```python
from build123d import *

# Parameters (mm, degrees)
SKETCH2_W             = 120
SKETCH2_H             = 160
SKETCH2_R             = 14.002160315
SKETCH2_R_2           = 1.35
BOSS_EXTRUDE1_DEPTH   = 4
SKETCH4_R             = 1.75
CUT_EXTRUDE1_DEPTH    = 4
SKETCH6_R             = 2.075123243
SKETCH6_R_2           = 1.889494125
BOSS_EXTRUDE2_DEPTH   = 4
BOSS_EXTRUDE2_2_DEPTH = 4
BOSS_EXTRUDE2_3_DEPTH = 4
BOSS_EXTRUDE2_4_DEPTH = 4


with BuildPart() as part:
    # Sketch2 → Boss-Extrude1 (new body)
    with BuildSketch(Plane(origin=(0, 0, 0), x_dir=(1, 0, 0), z_dir=(0, 1, 0))):
        Rectangle(SKETCH2_W, SKETCH2_H)
        Circle(SKETCH2_R, mode=Mode.SUBTRACT)
        with Locations((-28.228110793, -22.694220691)):
            Circle(SKETCH2_R_2, mode=Mode.SUBTRACT)
        with Locations((-24.5, -29)):
            Circle(SKETCH2_R_2, mode=Mode.SUBTRACT)
        with Locations((24.5, -29)):
            Circle(SKETCH2_R_2, mode=Mode.SUBTRACT)
        with Locations((29.771889207, -22.694220691)):
            Circle(SKETCH2_R_2, mode=Mode.SUBTRACT)
        with Locations((29.771889207, 26.305779309)):
            Circle(SKETCH2_R_2, mode=Mode.SUBTRACT)
        with Locations((24.5, 29)):
            Circle(SKETCH2_R_2, mode=Mode.SUBTRACT)
        with Locations((-28.228110793, 26.305779309)):
            Circle(SKETCH2_R_2, mode=Mode.SUBTRACT)
        with Locations((-24.5, 29)):
            Circle(SKETCH2_R_2, mode=Mode.SUBTRACT)
    extrude(amount=BOSS_EXTRUDE1_DEPTH)

    # Sketch4 → Cut-Extrude1 (cut)
    with BuildSketch(Plane(origin=(0, 4, 0), x_dir=(1, 0, 0), z_dir=(0, 1, 0))):
        with Locations((-6, 74.910885073)):
            Circle(SKETCH4_R)
        with Locations((-6, 69.410885073)):
            Circle(SKETCH4_R)
        with Locations((-55.5, 69.410885073)):
            Circle(SKETCH4_R)
        with Locations((-55.5, 74.910885073)):
            Circle(SKETCH4_R)
        with Locations((55.5, 74.910885073)):
            Circle(SKETCH4_R)
        with Locations((55.5, 69.410885073)):
            Circle(SKETCH4_R)
        with Locations((6, 69.410885073)):
            Circle(SKETCH4_R)
        with Locations((6, 74.910885073)):
            Circle(SKETCH4_R)
        with Locations((-6, -69)):
            Circle(SKETCH4_R)
        with Locations((-6, -74.5)):
            Circle(SKETCH4_R)
        with Locations((-55.5, -74.5)):
            Circle(SKETCH4_R)
        with Locations((-55.5, -69)):
            Circle(SKETCH4_R)
        with Locations((55.5, -69)):
            Circle(SKETCH4_R)
        with Locations((55.5, -74.5)):
            Circle(SKETCH4_R)
        with Locations((6, -74.5)):
            Circle(SKETCH4_R)
        with Locations((6, -69)):
            Circle(SKETCH4_R)
    extrude(amount=-CUT_EXTRUDE1_DEPTH, mode=Mode.SUBTRACT)


with BuildPart() as body_2:
    # Sketch6 → Boss-Extrude2 (new body)
    with BuildSketch(Plane(origin=(0, 4, 0), x_dir=(1, 0, 0), z_dir=(0, 1, 0))):
        with BuildLine():
            Line((60, 45), (60, 65))
            Line((60, 65), (60, 80))
            Line((60, 80), (85, 80))
            Line((85, 80), (85, 65))
            Line((85, 65), (80, 65))
            ThreePointArc((80, 65), (65.857864376, 59.142135624), (60, 45))
        make_face()
        with Locations((80.2, 72.5)):
            Circle(SKETCH6_R, mode=Mode.SUBTRACT)
        with Locations((65.5, 72.5)):
            Circle(SKETCH6_R_2, mode=Mode.SUBTRACT)
    extrude(amount=-BOSS_EXTRUDE2_DEPTH)


with BuildPart() as body_3:
    # Sketch6 → Boss-Extrude2 2 (new body)
    with BuildSketch(Plane(origin=(0, 4, 0), x_dir=(1, 0, 0), z_dir=(0, 1, 0))):
        with BuildLine():
            Line((-85, 80), (-85, 65))
            Line((-85, 65), (-80, 65))
            ThreePointArc((-80, 65), (-65.857864376, 59.142135624), (-60, 45))
            Line((-60, 45), (-60, 80))
            Line((-60, 80), (-85, 80))
        make_face()
        with Locations((-80.2, 72.5)):
            Circle(SKETCH6_R, mode=Mode.SUBTRACT)
        with Locations((-65.5, 72.5)):
            Circle(SKETCH6_R_2, mode=Mode.SUBTRACT)
    extrude(amount=-BOSS_EXTRUDE2_2_DEPTH)


with BuildPart() as body_4:
    # Sketch6 → Boss-Extrude2 3 (new body)
    with BuildSketch(Plane(origin=(0, 4, 0), x_dir=(1, 0, 0), z_dir=(0, 1, 0))):
        with BuildLine():
            Line((85, -80), (85, -65))
            Line((85, -65), (80, -65))
            ThreePointArc((80, -65), (65.857864376, -59.142135624), (60, -45))
            Line((60, -45), (60, -65))
            Line((60, -65), (60, -80))
            Line((60, -80), (85, -80))
        make_face()
        with Locations((65.5, -72.5)):
            Circle(SKETCH6_R_2, mode=Mode.SUBTRACT)
        with Locations((80.2, -72.5)):
            Circle(SKETCH6_R, mode=Mode.SUBTRACT)
    extrude(amount=-BOSS_EXTRUDE2_3_DEPTH)


with BuildPart() as body_5:
    # Sketch6 → Boss-Extrude2 4 (new body)
    with BuildSketch(Plane(origin=(0, 4, 0), x_dir=(1, 0, 0), z_dir=(0, 1, 0))):
        with BuildLine():
            Line((-60, -80), (-60, -45))
            ThreePointArc((-60, -45), (-65.857864376, -59.142135624), (-80, -65))
            Line((-80, -65), (-85, -65))
            Line((-85, -65), (-85, -80))
            Line((-85, -80), (-60, -80))
        make_face()
        with Locations((-65.5, -72.5)):
            Circle(SKETCH6_R_2, mode=Mode.SUBTRACT)
        with Locations((-80.2, -72.5)):
            Circle(SKETCH6_R, mode=Mode.SUBTRACT)
    extrude(amount=-BOSS_EXTRUDE2_4_DEPTH)


with BuildPart() as body_3_1:
    add(body_3.part)

    # Combine1: union part, body 2, body 4, body 5
    add(part.part)
    add(body_2.part)
    add(body_4.part)
    add(body_5.part)


solid = body_3_1.part
```
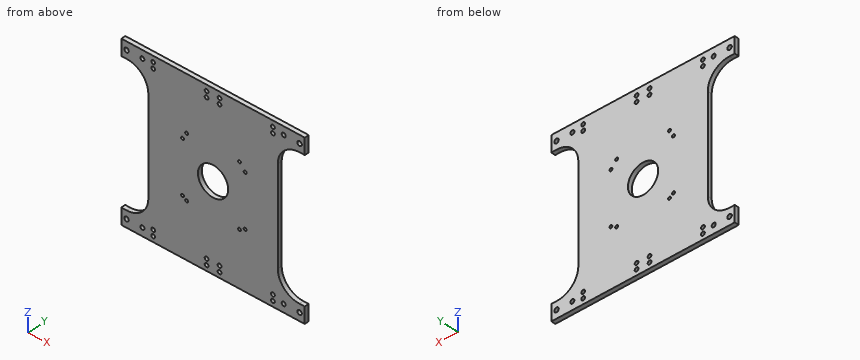
Input: part model. Units: mm. Frame: model coordinates. Round coordinates to 2 decimals unless told otherwise and drop trailing zeros. Write each loop counter-clockwise with the first axis right and the second up, starting at its lowest first coordinate (ties: lowest second). Pieces come first, ordered by that corner, then holes. Notation, with made-up numbers: (30, 81) -> (57, 81) arc R34 ccw to (57, 120) -> close; hole circle Ø4 at (75, -20). An arc over 180 degrees is marked (long way). Answer as CSV lines item,"result".
1. Section C-C (y = 1.15). Give the number of separate pieces and of enclosed holes in the cut face, plus the area to 3 significant figures.
Geometry says:
separate pieces,"1"
enclosed holes,"33"
area,"20,100 mm^2"
2. Section D-D (z = -16.5). Return the cut outline in (x, y), plus the area to 3 significant figures.
Geometry says:
outline,"(-60, 0) -> (60, 0) -> (60, 4) -> (-60, 4) -> close"
area,"480 mm^2"
3. Section A-A (z = 11). Return the cut outline in (x, y).
Geometry says:
outline,"(-60, 0) -> (-8.66, 0) -> (-8.66, 4) -> (-60, 4) -> close; (8.66, 0) -> (60, 0) -> (60, 4) -> (8.66, 4) -> close"
4. Section B-B (x = 2). Return the cut outline in (y, z).
Geometry says:
outline,"(0, -80) -> (4, -80) -> (4, -13.86) -> (0, -13.86) -> close; (0, 13.86) -> (4, 13.86) -> (4, 80) -> (0, 80) -> close"
5. Contact query for a flat-ended pin moving along its axis: P1, Ø1.5, axis at y = 1, z = 13.5, coming from the +X side. Output: stop coordinate, or through.
Geometry says:
P1,"stops at x = 60"
6. Ray query, L1, parallel to X at y = 2.1, z = 69; L2, parallel to X at y = 1.4, z = -26.5; L3, parallel to X at y = 1.75, z = -29. Return the intervals inside material, ascending. Write a range as [from, to].
Geometry says:
L1,"x = [-85, -57.25], [-53.75, -7.75], [-4.25, 4.25], [7.75, 53.75], [57.25, 85]"
L2,"x = [-60, -29.56], [-26.89, 28.44], [31.11, 60]"
L3,"x = [-60, -25.85], [-23.15, 23.15], [25.85, 60]"
